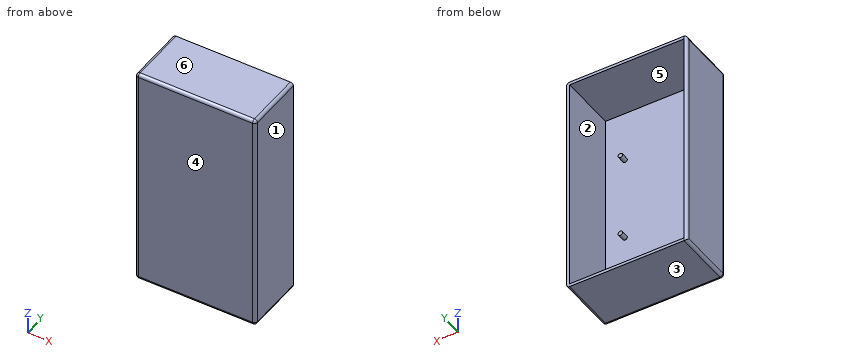
```python
from build123d import *

# Parameters (mm, degrees)
SKETCH1_W           = 80
SKETCH1_H           = 150
BOSS_EXTRUDE1_DEPTH = 40
SKETCH2_W           = 76
SKETCH2_H           = 146
CUT_EXTRUDE1_DEPTH  = 38
SKETCH4_R           = 1.5
BOSS_EXTRUDE3_DEPTH = 5
FILLET1_R           = 2


with BuildPart() as part:
    # Sketch1 → Boss-Extrude1 (new body)
    with BuildSketch(Plane(origin=(0, 0, 0), x_dir=(1, 0, 0), z_dir=(0, 1, 0))):
        with Locations((-8.86592033, 41.755152562)):
            Rectangle(SKETCH1_W, SKETCH1_H)
    extrude(amount=BOSS_EXTRUDE1_DEPTH)

    # Sketch2 → Cut-Extrude1 (cut)
    with BuildSketch(Plane(origin=(0, 40, 0), x_dir=(1, 0, 0), z_dir=(0, 1, 0))):
        with Locations((-8.86592033, 41.755152562)):
            Rectangle(SKETCH2_W, SKETCH2_H)
    extrude(amount=-CUT_EXTRUDE1_DEPTH, mode=Mode.SUBTRACT)

    # Sketch4 → Boss-Extrude3 (add)
    with BuildSketch(Plane(origin=(0, 2, 0), x_dir=(1, 0, 0), z_dir=(0, 1, 0))):
        with Locations(Location((-33.86592033, 60.072338785, 0), (0, 0, 270))):
            Circle(SKETCH4_R)
        with Locations(Location((-33.86592033, 3.072338785, 0), (0, 0, 270))):
            Circle(SKETCH4_R)
        with Locations(Location((16.13407967, 60.072338785, 0), (0, 0, 90))):
            Circle(SKETCH4_R)
        with Locations(Location((16.13407967, 3.072338785, 0), (0, 0, 90))):
            Circle(SKETCH4_R)
    extrude(amount=BOSS_EXTRUDE3_DEPTH)

    # Fillet1
    fillet1_edges = [part.edges().sort_by_distance(p)[0] for p in [
        (-48.86592033, 40, -41.755152562),
        (-8.86592033, 0, -116.755152562),
        (31.13407967, 0, -41.755152562),
        (-8.86592033, 0, 33.244847438),
        (-48.86592033, 0, -41.755152562),
        (-48.86592033, 20, -116.755152562),
        (31.13407967, 20, -116.755152562),
        (31.13407967, 20, 33.244847438),
        (-48.86592033, 20, 33.244847438),
    ]]
    fillet(fillet1_edges, radius=FILLET1_R - 0.0001)  # a hair under: the kernel refuses the full size


solid = part.part
```
Check sheet for the modelled part. Datum: model origin and axes. Units: mm. Face numbers are marked on the shaded views. A direction names the side the tool comes from. Coordinates: 2 decimals unless noted, no trailing zeros. Write each loop counter-clockwise with the first axis right and the second up, starting at its lowest first coordinate (ties: lowest second). Pieces come first, ordered by that corner, then holes. Notation, with made-up numbers: (5.5, 4) -> (11.5, 4) arc R29 cw to (11.5, 27) -> close; hole circle Ø4 at (67.5, -38.75). An arc over 180 degrees is marked (long way). Use a Markdown table: item, result.
1. Sectioned sample at D-D (x = -29). Enter the section's corners in (y, z).
Reported:
| item | result |
|---|---|
| outline | (0, -114.76) arc R2 ccw to (2, -116.76) -> (40, -116.76) -> (40, -114.76) -> (2, -114.76) -> (2, 31.24) -> (40, 31.24) -> (40, 33.24) -> (2, 33.24) arc R2 ccw to (0, 31.24) -> close |
2. Scan lines: line 1 along X through (y, z) = (24.5, -96); line 2 along Z through (x, y) = (-20.5, 10.5); line 3 along Y through (x, z) = (-10.5, 10). Record each from-to range of solid material in increasing order.
Reported:
| item | result |
|---|---|
| line 1 | x = -48.87 to -46.87, 29.13 to 31.13 |
| line 2 | z = -116.76 to -114.76, 31.24 to 33.24 |
| line 3 | y = 0 to 2 |
3. Go/stop test with flat-tipped pins: pin 1 Ø0.9 at (x, z) = (-34, -2.5) entering from +Y; pin 2 Ø3 at (x, z) = (20, -99) entering from +Y. Record where each tip stops, or that it passes through.
Reported:
| item | result |
|---|---|
| pin 1 | stops at y = 7 |
| pin 2 | stops at y = 2 |
4. Sectioned sample at A-A (y = 26). Enter the section's corners in (x, z).
Reported:
| item | result |
|---|---|
| outline | (-48.87, -114.76) arc R2 ccw to (-46.87, -116.76) -> (29.13, -116.76) arc R2 ccw to (31.13, -114.76) -> (31.13, 31.24) arc R2 ccw to (29.13, 33.24) -> (-46.87, 33.24) arc R2 ccw to (-48.87, 31.24) -> close; hole (-46.87, -114.76) -> (29.13, -114.76) -> (29.13, 31.24) -> (-46.87, 31.24) -> close |
5. Release check for a two-part mould opening along Z. For the marked faces 3, 4, 5 and 6 record: pulls with the +Z half, pulls with the -Z half, needs draft (parallel to the pull), parting line crosses it, or undercut.
Reported:
| item | result |
|---|---|
| face 3 | pulls with the -Z half |
| face 4 | needs draft |
| face 5 | undercut |
| face 6 | pulls with the +Z half |
6. Sectioned sample at B-B (y = 5.5). Enter the section's corners in (x, z), plus the area to 3 significant figures.
Reported:
| item | result |
|---|---|
| outline | (-48.87, -114.76) arc R2 ccw to (-46.87, -116.76) -> (29.13, -116.76) arc R2 ccw to (31.13, -114.76) -> (31.13, 31.24) arc R2 ccw to (29.13, 33.24) -> (-46.87, 33.24) arc R2 ccw to (-48.87, 31.24) -> close; circle Ø3 at (-33.87, -60.07); circle Ø3 at (-33.87, -3.07); circle Ø3 at (16.13, -60.07); circle Ø3 at (16.13, -3.07); hole (-46.87, -114.76) -> (29.13, -114.76) -> (29.13, 31.24) -> (-46.87, 31.24) -> close |
| area | 929 mm2 |
7. Tool access check on the marked faces 1 and 2. Record the directions out of +Z, -Z, +X, -X, +Y, -Y that give a thin tool (end or side, any length) a straight path to the whole face; none if there is none.
Reported:
| item | result |
|---|---|
| face 1 | +Z, -Z, +X, +Y, -Y |
| face 2 | +Y |
